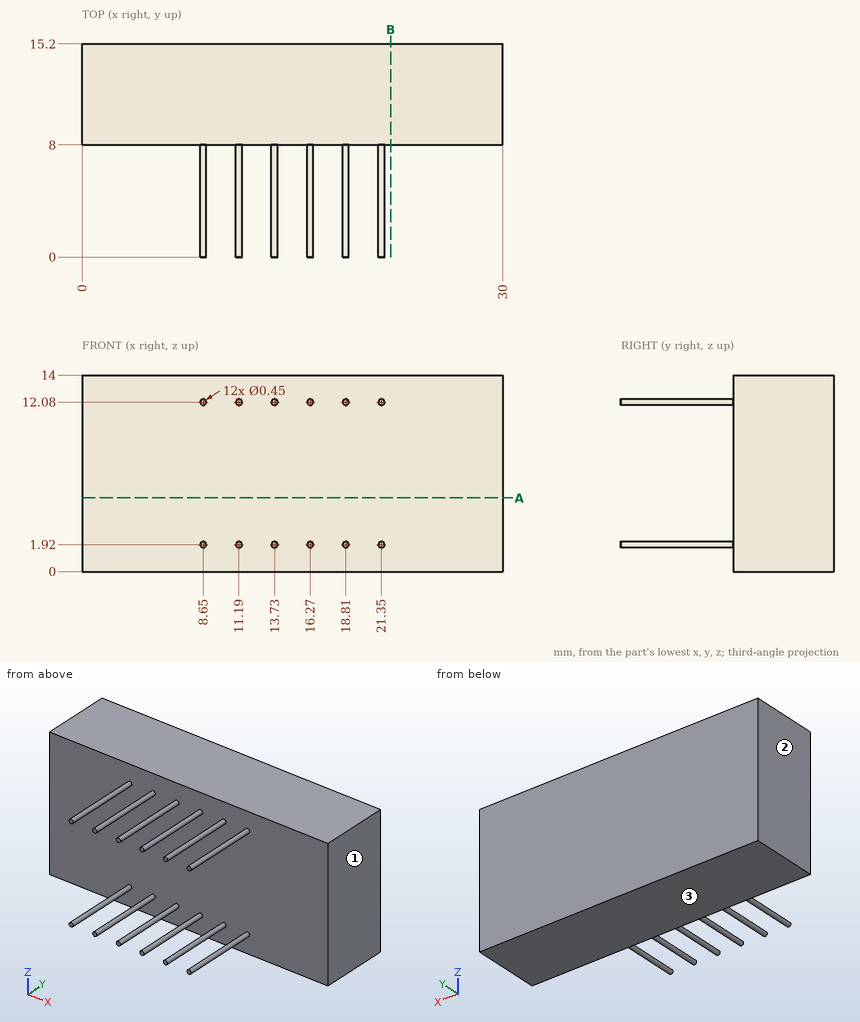
Geometry check sheet. Reference: drawing and pictorial views, mm from the part's lowest x, y, z. Give positions to 0.01 mm unless a question says otherwise; leave off trailing zeros. Order: outer loops, then holes, each group sorted by start corner. A loop starts at its lowest first (then second) coordinate and runs counter-clockwise, first axis right, second up. Notation, with made-up numbers: M 0,-9.5 L 36,-9.5 A38 ccw 36,29.5 Z; hole C -30,13.25 d7. An arc over 180 degrees is marked long. Answer in a Markdown table with one row per item. Add a question column.
Q1. Release check for a two-part mould opening along X. For the marked faces 1, 2 and 3 record: released by +X, released by -X, zero draft, split by the parting line, or undercut.
Q2. Thickness scan on L1, parallel to Y at x = 20, z = 6.75; L2, parallel to X at y = 3.25, z = 12. Record the ranges inside material, lowest first.
Q3. Sectioned sample at A-A, the plane z = 5.25. Record the boundary of the cut face in (x, y), and give its area (3 significant figures).
Q4. Sectioned sample at B-B, the plane x = 22. Record the boundary of the cut face in (y, z), and give its area (3 significant figures).
Q5. Gauge pin test, flat ends, axial feed: pin 1 Ø7 at (x, z) = (21.5, 6.5) entering from -Y; pin 2 Ø1.5 at (y, z) = (5.5, 6) entering from -X. Record the tip position at first contact, or that the pin passes through.
Verdict:
| question | item | result |
|---|---|---|
| 1 | face 1 | released by +X |
| 1 | face 2 | released by -X |
| 1 | face 3 | zero draft |
| 2 | L1 | 8 to 15.2 |
| 2 | L2 | 8.44 to 8.86, 10.98 to 11.4, 13.52 to 13.94, 16.06 to 16.48, 18.6 to 19.02, 21.14 to 21.56 |
| 3 | outline | M 0,8 L 30,8 L 30,15.2 L 0,15.2 Z |
| 3 | area | 216 mm² |
| 4 | outline | M 8,0 L 15.2,0 L 15.2,14 L 8,14 Z |
| 4 | area | 101 mm² |
| 5 | pin 1 | y = 8 |
| 5 | pin 2 | through |
